Work out the finished part from the listing and answer in its coordinate system (mm). Face numbers are marked on the shaded views. A direction names the side the tool comes from. Give positions to 0.01 mm unless a question says otherwise; leave off trailing zeros. Order: outer loops, then holes, each group sorted by start corner. A loop starts at its lowest first (then second) coordinate and runs counter-clockwise, first axis right, second up.
Autodesk Inventor part; units mm, degrees
ref_plane "YZ Plane" through (0, 0, 0) normal (1, 0, 0) x (0, 1, 0)
ref_plane "XZ Plane" through (0, 0, 0) normal (0, 1, 0) x (-1, 0, 0)
ref_plane "XY Plane" through (0, 0, 0) normal (0, 0, 1) x (1, 0, 0)
sketch "Sketch1" plane through (0, 0, 0) normal (1, 0, 0) x (0, 1, 0)
  line L0 (0, -2) -> (0, -40)
  line L1 (0, -40) -> (38, -40)
  line L2 (4, -2) -> (4, -36)
  line L3 (4, -36) -> (38, -36)
  line L4 (2, 0) -> (2, 0)
  line L5 (40, -38) -> (40, -38)
  arc A0 (40, -38) -> (38, -36) centre (38, -38) ccw
  arc A1 (38, -40) -> (40, -38) centre (38, -38) ccw
  arc A2 (4, -2) -> (2, 0) centre (2, -2) ccw
  arc A3 (2, 0) -> (0, -2) centre (2, -2) ccw
  point P0 (0, 0)
  point P1 (40, -40)
  point P2 (2, 0)
  dimension "d0" = 40
  dimension "d1" = 40
  dimension "d2" = 4
  dimension "d3" = 2
extrude "Extrusion1" add sketch "Sketch1" along normal blind 40
sketch "Sketch2" plane through (0, 4, -2) normal (0, 1, 0) x (1, 0, 0)
  line L0 (0, 34) -> (0, 0)
  line L1 (0, 0) -> (40, 0)
  line L2 (40, 34) -> (40, 0)
  line L3 (0, 34) -> (40, 34)
  point P0 (0, -2)
  point P1 (20, 17)
hole "Hole1" at (20, 4, -19) direction (0, -1, 0) diameter 10 end through all
sketch "Sketch3" plane through (0, 4, -36) normal (0, 0, 1) x (1, 0, 0)
  line L0 (0, 34) -> (0, 0) construction
  line L1 (0, 0) -> (40, 0) construction
  line L2 (40, 34) -> (40, 0) construction
  line L3 (0, 34) -> (40, 34) construction
  point P0 (0, -4)
  point P1 (20, 17)
hole "Hole2" at (20, 21, -36) direction (0, 0, -1) diameter 10 end through all
properties part number "LVas"
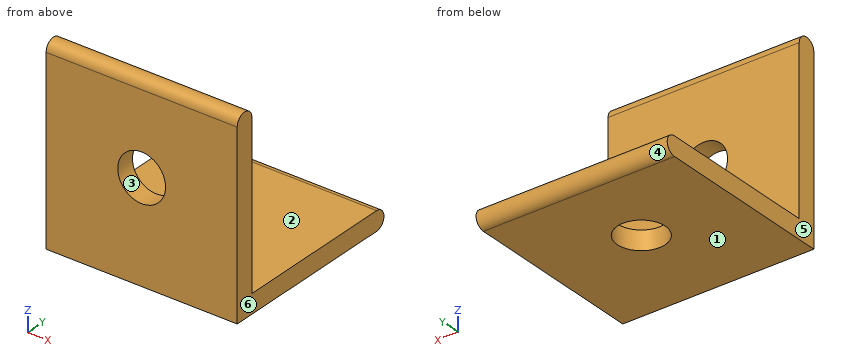
1. The part is cut by section B-B (z = -19). Write down the section's boundary in (x, y), then the cut area to 3 significant figures.
Findings below:
outline: (0, 0) - (15, 0) - (15, 4) - (0, 4) - close; (25, 0) - (40, 0) - (40, 4) - (25, 4) - close
area: 120 mm2
2. Which of the six approach directions +Z, -Z, +X, -X, +Y, -Y give full straight-line access (tool end or side, diameter ignored) to the marked faces 1 and 2?
Findings below:
face 1: -Z, +X, -X, +Y, -Y
face 2: +Z, +X, -X, +Y
3. The part is cut by section A-A (y = 21). Write down the section's boundary in (x, z), then the cut area to 3 significant figures.
Findings below:
outline: (0, -40) - (15, -40) - (15, -36) - (0, -36) - close; (25, -40) - (40, -40) - (40, -36) - (25, -36) - close
area: 120 mm2
4. The part is cut by section D-D (x = 6.5). Write down the section's boundary in (y, z), then the cut area to 3 significant figures.
Findings below:
outline: (0, -40) - (38, -40) arc R2 ccw to (38, -36) - (4, -36) - (4, -2) arc R2 ccw to (0, -2) - close
area: 301 mm2
5. Given P1, Ø8, axis at x = 20, z = -19, coming from the +Y side; P2, Ø6, axis at x = 7.5, y = 21.5, coming from the +Z side; P3, Ø12, axis at x = 30.5, z = -27, coming from the +Y side; P4, Ø3, axis at x = 34.5, z = -13.5, coming from the -Y side, each flat-ended and moving along its own axis, determine where each tip first touches the part or whether it passes through.
Findings below:
P1: passes through
P2: stops at z = -36
P3: stops at y = 4
P4: stops at y = 0
6. Straight lines are drawn through the part: probe 1 along Y at (x, z) = (20, -38.1); probe 2 along Y at (x, z) = (37.5, -22); probe 3 along X at (y, z) = (21, -38.15). For each, find the intervals that lie inside material, in ascending order.
Findings below:
probe 1: y = 0 to 16, 26 to 40
probe 2: y = 0 to 4
probe 3: x = 0 to 15, 25 to 40
7. The part is cut by section C-C (x = 20). Write down the section's boundary in (y, z).
Findings below:
outline: (0, -40) - (16, -40) - (16, -36) - (4, -36) - (4, -24) - (0, -24) - close; (0, -14) - (4, -14) - (4, -2) arc R2 ccw to (0, -2) - close; (26, -40) - (38, -40) arc R2 ccw to (38, -36) - (26, -36) - close
8. The mould has two halves that part along X. Classify the marked faces 3, 4, 5 and 6: pulls with the +X half, pulls with the -X half, needs draft (parallel to the pull), parting line crosses it, or undercut.
Findings below:
face 3: undercut
face 4: needs draft
face 5: pulls with the -X half
face 6: pulls with the +X half
